Can you work these out from the drawing? Everything is in mm from the part's minimum corner. A direction names the side the tool comes from. Coordinates: 2 decimals unless noted, no trailing zeros. Write each loop counter-clockwise with the first axis right and the second up, starting at its lowest first coordinate (ties: lowest second). Pieces come first, ordered by that corner, then holes.
(1) Please list where these lines run through material, in increasing order: probe 1 along Z at (x, y) = (17.5, 278); probe 2 along Y at (x, z) = (3.25, 47); probe 3 along Y at (x, z) = (16, 68).
(2) Imagine slicing it at C-C, the plane y = 124. List the corners of the cut face in (x, z) for me, plus the area to 3 significant figures.
(3) For pin 1 Ø2 at (x, y) = (9, 94.5) entering from +Z; pin 2 Ø5 at (x, y) = (17.5, 197) entering from -Z; pin 3 Ø6 at (x, z) = (22, 19) entering from -Y, each with a flat end and sliding along its axis, tell me the tip position at first contact or that it passes through.
(4) Which directions (+Z, -Z, +X, -X, +Y, -Y) give clear straight access to the entire face, cutting with the end or side of a thin tool? Please do the marked faces 1, 2 and 3.
(5) Imagine slicing it at A-A, the plane x = 15. List the corners of the cut face in (y, z) for me, plus the area to 4 significant figures.
(6) Imagine slicing it at D-D, the plane z = 9. List the corners of the cut face in (x, y) for me, plus the area to 3 significant figures.
(7) Imagine slicing it at B-B, the plane z = 62.5. List the corners of the cut face in (x, y) for me, plus the area to 3 significant figures.
(8) Thinking about a two-plate mould opening in Z: for the marked faces 4, 5, 6 and 7, which applies, released by +Z, released by -Z, zero draft, split by the parting line, or undercut?
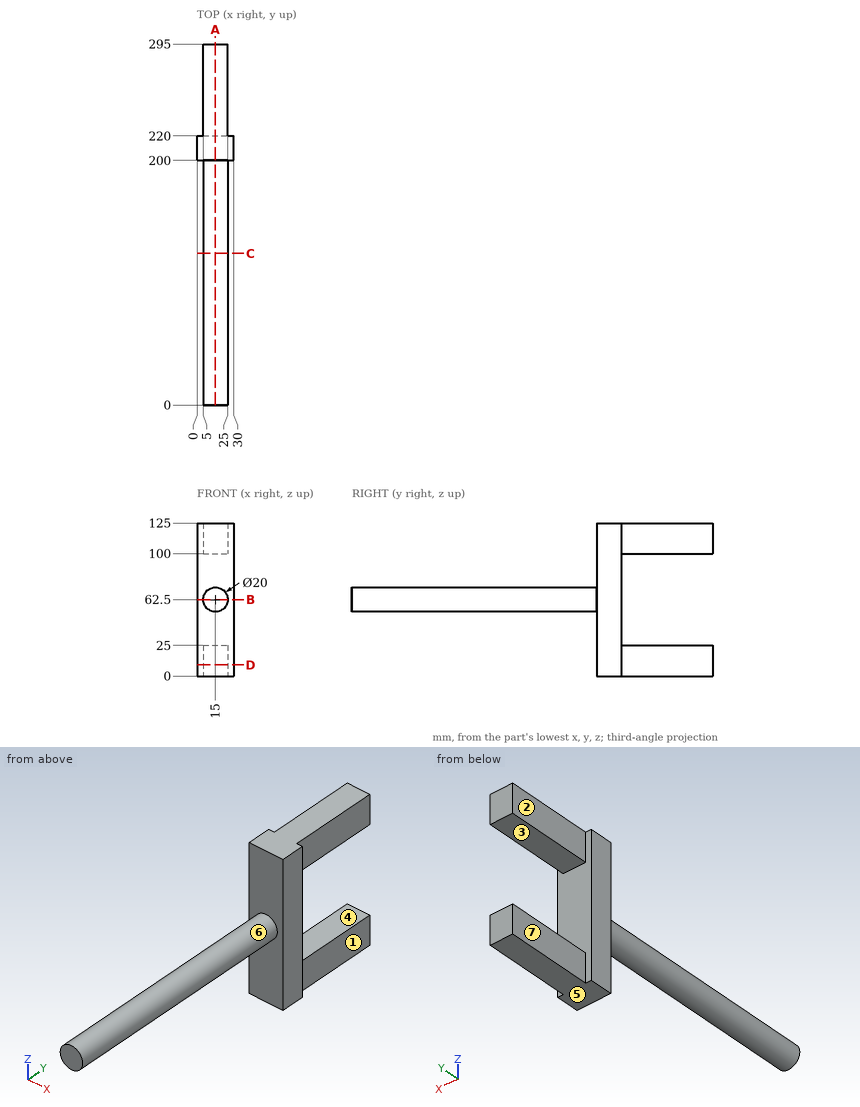
Recorded:
1. probe 1: z = 0 to 25, 100 to 125
1. probe 2: y = 200 to 220
1. probe 3: y = 0 to 220
2. outline: circle Ø20 at (15, 62.5)
2. area: 314 mm2
3. pin 1: stops at z = 71.16
3. pin 2: stops at z = 52.5
3. pin 3: stops at y = 200
4. face 1: +Z, -Z, +X, +Y
4. face 2: +Z, -Z, -X, +Y
4. face 3: +X, -X, +Y
5. outline: (0, 52.5) - (200, 52.5) - (200, 0) - (295, 0) - (295, 25) - (220, 25) - (220, 100) - (295, 100) - (295, 125) - (200, 125) - (200, 72.5) - (0, 72.5) - close
5. area: 10,250 mm2
6. outline: (0, 200) - (30, 200) - (30, 220) - (25, 220) - (25, 295) - (5, 295) - (5, 220) - (0, 220) - close
6. area: 2,100 mm2
7. outline: (0, 200) - (5, 200) - (5, 0) - (25, 0) - (25, 200) - (30, 200) - (30, 220) - (0, 220) - close
7. area: 4,600 mm2
8. face 4: undercut
8. face 5: released by -Z
8. face 6: split by the parting line
8. face 7: zero draft
